Work out the finished part from the listing and answer in its coordinate system (mm). Round coordinates to 2 decimals unless told otherwise and drop trailing zeros. Write each loop counter-clockwise with the first axis right and the second up, starting at its lowest first coordinate (ties: lowest second). Pieces come first, ordered by that corner, then holes.
1. A flat-ended cylindrical pin translates along its axis: pin 1 Ø1 at (x, z) = (2.5, 1.5) entering from -Y. Find the tip coordinate at first contact, or state that the pin passes through.
2. Straight lines are drawn through the part: probe 1 along Z at (x, y) = (3, -7.5); probe 2 along Z at (x, y) = (1.7, -6.75); probe 3 along Z at (x, y) = (0.6, -1). For each, find the intervals that lie inside material, in ascending order.
3. Determine the mould class of faces 1 (the face through (0, 3, 0)), 2 (the face through (1.6, -11.4, -23.812)), 3 (the face through (1.565, -6.865, 17.879)) for opening direction Z: pulls with the +Z half, pulls with the -Z half, needs draft (parallel to the pull), parting line crosses it, or undercut.
4. Find section A-A (z = 0). Write down the section's boundary in (x, y) (3 decimals), and give its area (3 significant figures).
5. Find section C-C (y = 7.25). Write down the section's boundary in (x, z) (3 decimals).
6. Find section B-B (x = 2.4). Write down the section's boundary in (y, z) (1 decimal), and give its area (3 significant figures).
```python
from build123d import *

# Parameters (mm, degrees)
SKETCH1_W                        = 47.625
SKETCH1_H                        = 23.8125
BOSS_EXTRUDE1_DEPTH              = 3.175
SKETCH2_R                        = 14.2875
CUT_EXTRUDE1_DEPTH               = 27.811836385
F_1_8_0_125_DIAMETER_HOLE1_D     = 3.175
F_1_8_0_125_DIAMETER_HOLE1_DEPTH = 19.001994
F_1_8_0_125_DIAMETER_HOLE1_TIP   = 0.953866233
FILLET1_R                        = 22.86


with BuildPart() as part:
    # Sketch1 → Boss-Extrude1 (new body)
    with BuildSketch(Plane(origin=(0, 0, 0), x_dir=(0, 0, -1), z_dir=(1, 0, 0))):
        Rectangle(SKETCH1_W, SKETCH1_H)
    extrude(amount=BOSS_EXTRUDE1_DEPTH)

    # Sketch2 → Cut-Extrude1 (cut, through all)
    with BuildSketch(Plane(origin=(3.175, 0, 0), x_dir=(0, 0, -1), z_dir=(1, 0, 0))):
        with Locations((0, -12.16025)):
            Circle(SKETCH2_R)
    extrude(amount=-CUT_EXTRUDE1_DEPTH, mode=Mode.SUBTRACT)

    # 1/8 (0.125) Diameter Hole1
    with Locations(Plane(origin=(3.175, 0, 0), x_dir=(0, 0, -1), z_dir=(1, 0, 0))):
        with Locations((-19.048871022, -7.9375), (0, 7.9375), (19.048871022, -7.9375)):
            Hole(F_1_8_0_125_DIAMETER_HOLE1_D / 2, depth=F_1_8_0_125_DIAMETER_HOLE1_DEPTH)
            with Locations((0, 0, -(F_1_8_0_125_DIAMETER_HOLE1_DEPTH + F_1_8_0_125_DIAMETER_HOLE1_TIP / 2))):  # 118° drill point
                Cone(0, F_1_8_0_125_DIAMETER_HOLE1_D / 2, F_1_8_0_125_DIAMETER_HOLE1_TIP, mode=Mode.SUBTRACT)

    # Fillet1
    fillet1_edges = [part.edges().sort_by_distance(p)[0] for p in [
        (1.5875, 11.90625, 23.8125),
        (1.5875, 11.90625, -23.8125),
    ]]
    fillet(fillet1_edges, radius=FILLET1_R)


solid = part.part
```
Worked answers:
1. pin 1: stops at y = 1.99
2. probe 1: z = -23.55 to -20.57, -17.52 to -13.51, 13.51 to 17.52, 20.57 to 23.55
2. probe 2: z = -23.42 to -20.1, -18 to -13.22, 13.22 to 18, 20.1 to 23.42
2. probe 3: z = -21.53 to -8.92, 8.92 to 21.53
3. face 1: needs draft
3. face 2: pulls with the -Z half
3. face 3: undercut
4. outline: (0, 2.127) - (3.175, 2.127) - (3.175, 6.35) - (0, 6.35) - close; (0, 9.525) - (3.175, 9.525) - (3.175, 11.906) - (0, 11.906) - close
4. area: 21.0 mm2
5. outline: (0, -14.78) - (3.175, -14.78) - (3.175, -1.431) - (0, -1.431) - close; (0, 1.431) - (3.175, 1.431) - (3.175, 14.78) - (0, 14.78) - close
6. outline: (-11.9, -23.8) - (-11, -23.8) arc R22.9 ccw to (11.9, -1) - (11.9, 1) arc R22.9 ccw to (-11, 23.8) - (-11.9, 23.8) - (-11.9, 14.3) arc R14.3 cw to (-11.9, -14.3) - close; hole circle Ø3.2 at (-7.9, -19); hole circle Ø3.2 at (-7.9, 19); hole circle Ø3.2 at (7.9, 0)
6. area: 573 mm2
